Check sheet for the modelled part. Datum: model origin and axes. Units: mm. Round coordinates to 2 decimals unless told otherwise and drop trailing zeros. Write each loop counter-clockwise with the first axis right and the second up, starting at its lowest first coordinate (ties: lowest second). Pieces come first, ordered by that corner, then holes. Notation, with made-up numbers: (73.5, -7.75) -> (82.5, -7.75) arc R20 ccw to (82.5, 6.25) -> close; hole circle Ø10 at (-38.5, 29.25). An arc over 180 degrees is marked (long way). Write item = value, one per line.
from build123d import *

# Parameters (mm, degrees)
SKETCH_W   = 43
SKETCH_H   = 30
SKETCH_R   = 5.25
SKETCH_R_2 = 1.6
PAD_DEPTH  = 2
FILLET_R   = 5


with BuildPart() as part:
    # Sketch → Pad (new body)
    with BuildSketch(Plane.XY):
        with Locations((21.5, 15)):
            Rectangle(SKETCH_W, SKETCH_H)
        with Locations((14.474775, 21.974684)):
            Circle(SKETCH_R, mode=Mode.SUBTRACT)
        with Locations((28.474684, 22.025225)):
            Circle(SKETCH_R, mode=Mode.SUBTRACT)
        with Locations((14.525316, 7.974775)):
            Circle(SKETCH_R, mode=Mode.SUBTRACT)
        with Locations((28.525225, 8.025316)):
            Circle(SKETCH_R, mode=Mode.SUBTRACT)
        with Locations((21.5, 15)):
            Circle(SKETCH_R_2, mode=Mode.SUBTRACT)
        with Locations((3.5, 15)):
            Circle(SKETCH_R_2, mode=Mode.SUBTRACT)
        with Locations((39.5, 15)):
            Circle(SKETCH_R_2, mode=Mode.SUBTRACT)
    extrude(amount=PAD_DEPTH)

    # Fillet
    fillet_edges = [part.edges().sort_by_distance(p)[0] for p in [
        (43, 0, 1),
        (43, 30, 1),
        (0, 0, 1),
        (0, 30, 1),
    ]]
    fillet(fillet_edges, radius=FILLET_R)


solid = part.part
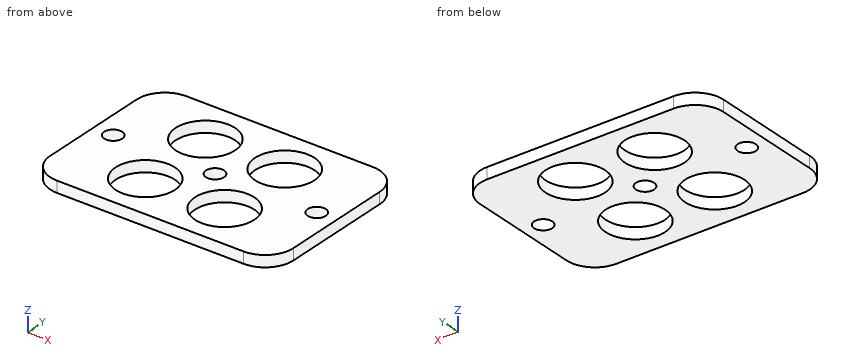
(1) Material ranges on L1, parallel to X at y = 21.75, z = 1.7; L2, parallel to Y at x = 21.5, z = 1.5; L3, parallel to X at y = 24.75, z = 1.2, recorded low to high. Write a range as [from, to].
Worked answers:
L1 = [0, 9.23], [19.72, 23.23], [33.72, 43]
L2 = [0, 13.4], [16.6, 30]
L3 = [0, 10.02], [18.93, 23.99], [32.96, 43]
(2) Sectioned sample at C-C on y = 24. Enter the section's corners in (x, z), then the cut area to 3 significant figures.
Worked answers:
outline = (0, 0) -> (9.63, 0) -> (9.63, 2) -> (0, 2) -> close; (19.32, 0) -> (23.61, 0) -> (23.61, 2) -> (19.32, 2) -> close; (33.34, 0) -> (43, 0) -> (43, 2) -> (33.34, 2) -> close
area = 47.2 mm²
(3) Sectioned sample at B-B on x = 14. Enter the section's corners in (y, z), then the cut area to 3 significant figures.
Worked answers:
outline = (0, 0) -> (2.75, 0) -> (2.75, 2) -> (0, 2) -> close; (13.2, 0) -> (16.75, 0) -> (16.75, 2) -> (13.2, 2) -> close; (27.2, 0) -> (30, 0) -> (30, 2) -> (27.2, 2) -> close
area = 18.2 mm²
(4) Go/stop test with flat-tipped pins: P1, Ø3, axis at x = 3.5, y = 15, coming from the -Z side; P2, Ø10, axis at x = 12, y = 11, coming from the +Z side. Record where each tip stops, or that it passes through.
Worked answers:
P1 = through
P2 = 2
(5) Sectioned sample at D-D on x = 3.5. Enter the section's corners in (y, z).
Worked answers:
outline = (0.23, 0) -> (13.4, 0) -> (13.4, 2) -> (0.23, 2) -> close; (16.6, 0) -> (29.77, 0) -> (29.77, 2) -> (16.6, 2) -> close
(6) Sectioned sample at A-A on y = 15. Enter the section's corners in (x, z), then the cut area to 3 significant figures.
Worked answers:
outline = (0, 0) -> (1.9, 0) -> (1.9, 2) -> (0, 2) -> close; (5.1, 0) -> (19.9, 0) -> (19.9, 2) -> (5.1, 2) -> close; (23.1, 0) -> (37.9, 0) -> (37.9, 2) -> (23.1, 2) -> close; (41.1, 0) -> (43, 0) -> (43, 2) -> (41.1, 2) -> close
area = 66.8 mm²
